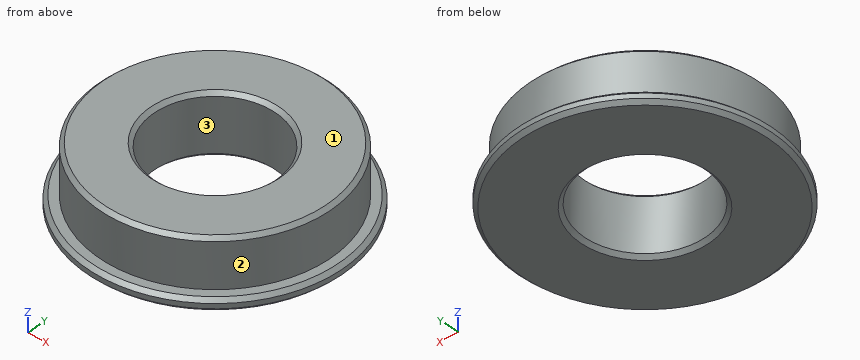
from build123d import *

# Parameters (mm, degrees)
SKETCH_1_R      = 9.5
SKETCH_1_R_2    = 5
EXTRUDE_1_DEPTH = 5
SKETCH_2_R      = 10.5
SKETCH_2_R_2    = 9.5
EXTRUDE_2_DEPTH = 1
CHAMFER_1_SIZE  = 0.3


with BuildPart() as part:
    # 草图1 → 凸台-拉伸1 (new body)
    with BuildSketch(Plane.XY):
        Circle(SKETCH_1_R)
        Circle(SKETCH_1_R_2, mode=Mode.SUBTRACT)
    extrude(amount=EXTRUDE_1_DEPTH)

    # 草图2 → 凸台-拉伸2 (add)
    with BuildSketch(Plane(origin=(0, 0, 0), x_dir=(-1, 0, 0), z_dir=(0, 0, -1))):
        Circle(SKETCH_2_R)
        Circle(SKETCH_2_R_2, mode=Mode.SUBTRACT)
    extrude(amount=-EXTRUDE_2_DEPTH)

    # 倒角1
    chamfer_1_edges = [part.edges().sort_by_distance(p)[0] for p in [
        (10.5, 0, 1),
        (10.5, 0, 0),
        (-9.5, 0, 5),
        (-5, 0, 0),
        (-5, 0, 5),
    ]]
    chamfer(chamfer_1_edges, length=CHAMFER_1_SIZE)


solid = part.part
Work out the finished part from the listing and answer in its coordinate system (mm). Face numbers are marked on the shaded views. Coordinates: 2 decimals unless noted, no trailing zeros. Loops run counter-clockwise (first coordinate to the right, second up) from the corner with the lowest first, then second, coordinate; pieces in that order, holes last. Notation, with made-up numbers: M -29.75,-34 L 19.25,-34 A29 cw 19.25,-4 Z; hole C 80.25,87.5 d1. An arc over 180 degrees is marked long. Answer in a Markdown table with one row per item. Add a question column.
1. Flat-ended cylindrical pins translate along their axes: P1, Ø1, axis at x = 7.5, z = 4, coming from the +Y side; P2, Ø1, axis at x = 6, z = 2.5, coming from the +Y side. Find the tip coordinate at first contact, or state that the pin passes through.
2. Consider L1, parallel to Y at x = 0, z = 3.35; L2, parallel to Y at x = 1.25, z = 2.4; L3, parallel to Z at x = -9.5, y = 1.5. Determine where each line is inside the solid, lowest interval first.
3. The mould has two halves that part along Y. Classify the marked faces 1, 2 and 3: pulls with the +Y half, pulls with the -Y half, needs draft (parallel to the pull), parting line crosses it, or undercut.
4. Find section A-A, the plane x = 0. Write down the section's boundary in (y, z), then the cut area to 4 significant figures.
Reported:
| question | item | result |
|---|---|---|
| 1 | P1 | stops at y = 6.42 |
| 1 | P2 | stops at y = 7.75 |
| 2 | L1 | y = -9.5 to -5, 5 to 9.5 |
| 2 | L2 | y = -9.42 to -4.84, 4.84 to 9.42 |
| 2 | L3 | z = 0 to 1 |
| 3 | face 1 | needs draft |
| 3 | face 2 | parting line crosses it |
| 3 | face 3 | undercut |
| 4 | outline | M -10.5,0.3 L -10.2,0 L -5.3,0 L -5,0.3 L -5,4.7 L -5.3,5 L -9.2,5 L -9.5,4.7 L -9.5,1 L -10.2,1 L -10.5,0.7 Z; M 5,0.3 L 5.3,0 L 10.2,0 L 10.5,0.3 L 10.5,0.7 L 10.2,1 L 9.5,1 L 9.5,4.7 L 9.2,5 L 5.3,5 L 5,4.7 Z |
| 4 | area | 46.55 mm^2 |
